The model under review builds one solid part; all positions refer to its coordinate system, in mm. Face numbers are marked on the shaded views. A direction names the side the tool comes from. Round coordinates to 2 decimals unless told otherwise and drop trailing zeros. Order: outer loops, then holes, each group sorted by start corner. A loop starts at its lowest first (then second) coordinate and runs counter-clockwise, first axis right, second up. Notation, with made-up numbers: M 7.25,-15 L 37.25,-15 A27 cw 37.25,1 Z; hole C -20,26.25 d10. An arc over 180 degrees is marked long. Use a Markdown table: item, result. Add a question column.
1. Consider section A-A on z = 17.5. State the section outline as (x, y) points, then the cut area to 3 significant figures.
2. Consider section B-B on z = 0.5. State the section outline as (x, y) points.
3. To check wall thickness, follow probe 1 along X at (y, z) = (5, 28.35); probe 2 along Z at (x, y) = (0, -3.75). State the ranges of each line that lie inside material, in increasing order.
4. Insertion check: P1, Ø4, axis at y = -0.5, z = -3.5, coming from the -X side; P2, Ø1.6, axis at x = 4.5, y = 4.5, coming from the -Z side; P3, Ø1.8, axis at x = 5, y = -5, coming from the +Z side; P4, Ø2, axis at x = -5, y = 4.5, coming from the +Z side. Each pin has a flat end and moves straight along its axis. Give the tip position at first contact, or say it passes through.
5. For the marked faces 1 and 2, list the 3-axis set-ups (+Z, -Z, +X, -X, +Y, -Y) from which the entire face can be reached by the end or side of a thin tool; tool diameter is ignored.
6. Consider section C-C on x = 0. State the section outline as (y, z) points.
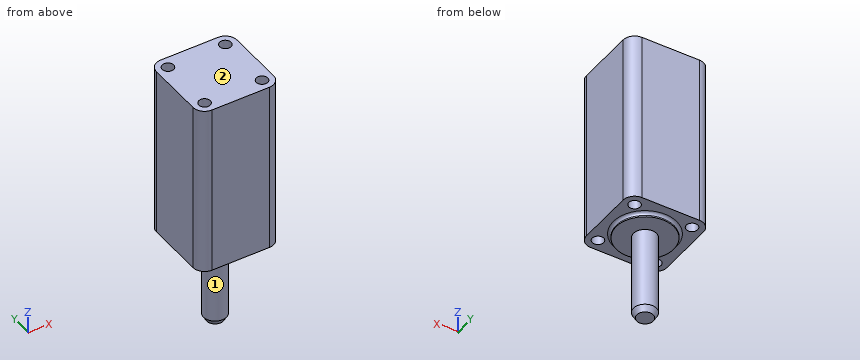
Autodesk Inventor part; units mm, degrees
ref_plane "YZ Plane" through (0, 0, 0) normal (1, 0, 0) x (0, 1, 0)
ref_plane "XZ Plane" through (0, 0, 0) normal (0, 1, 0) x (-1, 0, 0)
ref_plane "XY Plane" through (0, 0, 0) normal (0, 0, 1) x (1, 0, 0)
sketch "Szkic1" plane through (0, 0, 0) normal (0, 0, 1) x (1, 0, 0)
  line L0 (7, -7) -> (-7, -7)
  line L1 (-7, -7) -> (-7, 7)
  line L2 (-7, 7) -> (7, 7)
  line L3 (7, 7) -> (7, -7)
  line L4 (7, -7) -> (-7, 7) construction
  line L5 (-7, -7) -> (7, 7) construction
  line L6 (0, 0) -> (-5.75, 0)
  line L7 (-7, 5.75) -> (-5, 5.75)
  line L8 (-5, 7) -> (-5, 5)
  line L9 (-5, 5) -> (5, 5)
  line L10 (5, 5) -> (5, -5)
  line L11 (5, -5) -> (-5, -5)
  line L12 (-5, -5) -> (-5, 5)
  circle A0 centre (-5, 5) radius 1
  circle A1 centre (5, 5) radius 1
  circle A2 centre (5, -5) radius 1
  circle A3 centre (-5, -5) radius 1
  circle A4 centre (0, 0) radius 5
  circle A5 centre (0, 0) radius 5.5
  circle A6 centre (0, 0) radius 2
  circle A7 centre (0, 0) radius 2.1
  dimension "d0" = 14
  dimension "d1" = 14
  dimension "d8" = 2
  dimension "d9" = 2
  dimension "d13" = 10
  dimension "d14" = 10
  dimension "d15" = 10
  dimension "d17" = 2
  dimension "d18" = 2
  dimension "d19" = 2
  dimension "d20" = 2
  dimension "d21" = 11
  dimension "d22" = 4
  dimension "d23" = 4.2
extrude "Wyciągnięcie proste1" add sketch "Szkic1" along normal blind 30 contours L0 L1 L7 A0 L12 A5 A3 L11 A2 L10 A1 L9 L8 L2 L3 | L1 L2 L8 A0 L7 | A0 L9 A5 L12 | A5 L9 A4 L12 | L12 L6 A5 | A5 L9 | A6 | A7 | L12 A5 L6 | A4 L11 A5 L12 | A4 | L9 A5 L10 A4 | L9 A1 L10 A5 | A5 L11 A3 L12 | A4 L10 A5 L11 | L11 A5 | L10 A5 | A5 L10 A2 L11
sketch "Szkic2" plane through (0, 0, 0) normal (0, 0, -1) x (-1, 0, 0)
  line L0 (7, -7) -> (-7, -7)
  line L1 (-7, -7) -> (-7, 7)
  line L2 (-7, 7) -> (7, 7)
  line L3 (7, 7) -> (7, -7)
  line L4 (7, -7) -> (-7, 7) construction
  line L5 (-7, -7) -> (7, 7) construction
  line L6 (0, 0) -> (-5.75, 0)
  line L7 (-7, 5.75) -> (-5, 5.75)
  line L8 (-5, 7) -> (-5, 5)
  line L9 (-5, 5) -> (5, 5)
  line L10 (5, 5) -> (5, -5)
  line L11 (5, -5) -> (-5, -5)
  line L12 (-5, -5) -> (-5, 5)
  circle A0 centre (-5, 5) radius 1
  circle A1 centre (5, 5) radius 1
  circle A2 centre (5, -5) radius 1
  circle A3 centre (-5, -5) radius 1
  circle A4 centre (0, 0) radius 5
  circle A5 centre (0, 0) radius 5.5
  circle A6 centre (0, 0) radius 2
  circle A7 centre (0, 0) radius 2.1
  dimension "d26" = 14
  dimension "d27" = 14
  dimension "d28" = 2
  dimension "d29" = 2
  dimension "d30" = 10
  dimension "d31" = 10
  dimension "d32" = 10
  dimension "d33" = 2
  dimension "d34" = 2
  dimension "d35" = 2
  dimension "d36" = 2
  dimension "d37" = 11
  dimension "d38" = 4
  dimension "d39" = 4.2
extrude "Wyciągnięcie proste2" add sketch "Szkic2" along normal blind 0.75 contours A6 | A7 | A4
fillet "Zaokrąglenie1" radius 2 4 edges at (-7, 7, 15) (7, 7, 15) (7, -7, 15) (-7, -7, 15)
fillet "Zaokrąglenie2" radius 0.5 1 edges at (5, 0, 0)
sketch "Szkic3" plane through (0, 0, -0.75) normal (0, 0, -1) x (-1, 0, 0)
  circle A0 centre (0, 0) radius 2
  dimension "d44" = 4
extrude "Wyciągnięcie proste3" add sketch "Szkic3" along normal blind 15
chamfer "Faza1" distance 1 angle 30 1 edges at (2, 0, -15.75) measured on face at (-1.9935, -0.1609, -10.75)
sketch "Szkic4" plane through (0, 0, 0) normal (0, 0, -1) x (-1, 0, 0)
  circle A0 centre (-5, 5) radius 1
  circle A1 centre (-5, 5) radius 1
  circle A2 centre (5, 5) radius 1
  circle A3 centre (5, 5) radius 1
  circle A4 centre (5, -5) radius 1
  circle A5 centre (5, -5) radius 1
  circle A6 centre (-5, -5) radius 1
  point P0 (0, 0)
extrude "Wyciągnięcie proste4" add sketch "Szkic4" against normal blind 26.8
sketch "Szkic5" plane through (0, 0, 0) normal (0, 0, -1) x (-1, 0, 0)
  circle A0 centre (-5, 5) radius 1
  circle A1 centre (-5, 5) radius 1
  circle A2 centre (5, 5) radius 1
  circle A3 centre (5, 5) radius 1
  circle A4 centre (5, -5) radius 1
  circle A5 centre (5, -5) radius 1
  circle A6 centre (-5, -5) radius 1
  circle A7 centre (-5, -5) radius 1
  point P0 (0, 0)
extrude "Wyciągnięcie proste5" cut sketch "Szkic5" against normal blind 3.2
properties part number "Silnik krokowy"
Answer block:
| question | item | result |
|---|---|---|
| 1 | outline | M -7,-5 A2 ccw -5,-7 L 5,-7 A2 ccw 7,-5 L 7,5 A2 ccw 5,7 L -5,7 A2 ccw -7,5 Z |
| 1 | area | 193 mm^2 |
| 2 | outline | M -7,-5 A2 ccw -5,-7 L 5,-7 A2 ccw 7,-5 L 7,5 A2 ccw 5,7 L -5,7 A2 ccw -7,5 Z; hole C -5,-5 d2; hole C -5,5 d2; hole C 5,-5 d2; hole C 5,5 d2 |
| 3 | probe 1 | -7 to -6, -4 to 4, 6 to 7 |
| 3 | probe 2 | -0.75 to 30 |
| 4 | P1 | x = -2 |
| 4 | P2 | z = 0 |
| 4 | P3 | z = 26.8 |
| 4 | P4 | z = 30 |
| 5 | face 1 | -Z |
| 5 | face 2 | +Z, +X, -X, +Y, -Y |
| 6 | outline | M -7,0 L -5.5,0 A0.5 cw -5,-0.5 L -5,-0.75 L -2,-0.75 L -2,-14.75 L -1.42,-15.75 L 1.42,-15.75 L 2,-14.75 L 2,-0.75 L 5,-0.75 L 5,-0.5 A0.5 cw 5.5,0 L 7,0 L 7,30 L -7,30 Z |
